```python
from build123d import *

# Parameters (mm, degrees)
SZKIC1_R                    = 6
SZKIC1_R_2                  = 3.5
DODANIE_WYCI_GNI_CIE1_DEPTH = 40
ZAOKR_GLENIE1_R             = 0.5
ZAOKR_GLENIE2_R             = 0.5


with BuildPart() as part:
    # Szkic1 → Dodanie-wyciągnięcie1 (new body)
    with BuildSketch(Plane.XY):
        Circle(SZKIC1_R)
        Circle(SZKIC1_R_2, mode=Mode.SUBTRACT)
    extrude(amount=-DODANIE_WYCI_GNI_CIE1_DEPTH)

    # Zaokrąglenie1
    zaokr_glenie1_edges = [part.edges().sort_by_distance(p)[0] for p in [
        (-6, 0, 0),
        (-6, 0, -40),
    ]]
    fillet(zaokr_glenie1_edges, radius=ZAOKR_GLENIE1_R)

    # Zaokrąglenie2
    zaokr_glenie2_edges = [part.edges().sort_by_distance(p)[0] for p in [
        (-3.5, 0, -40),
        (-3.5, 0, 0),
    ]]
    fillet(zaokr_glenie2_edges, radius=ZAOKR_GLENIE2_R)


solid = part.part
```
CAD build for the part. Positions are in the model's coordinates, mm. Give positions to 0.01 mm unless a question says otherwise; leave off trailing zeros. Loops run counter-clockwise (first coordinate to the right, second up) from the corner with the lowest first, then second, coordinate; pieces in that order, holes last. Notation, with made-up numbers: (13, 36.5) - (29, 36.5) arc R21 ccw to (29, 41.5) - close; hole circle Ø1 at (68.25, 73). An arc over 180 degrees is marked (long way). Put each result on its own line as item: value.
Q1. Mould opens along Y. For faces 1 (the face through (3.233, -1.341, -19.727)), 2 (the face through (-4, -2, -40)), 3 (the face through (-6, 0, -20)) say: pulls with the +Y half, pulls with the -Y half, needs draft (parallel to the pull), parting line crosses it, or undercut.
Filled in:
face 1: undercut
face 2: needs draft
face 3: parting line crosses it
Q2. Slice it at A-A (x = 0). Give the cut face in (y, z).
Filled in:
outline: (-6, -39.5) arc R0.5 ccw to (-5.5, -40) - (-4, -40) arc R0.5 ccw to (-3.5, -39.5) - (-3.5, -0.5) arc R0.5 ccw to (-4, 0) - (-5.5, 0) arc R0.5 ccw to (-6, -0.5) - close; (3.5, -39.5) arc R0.5 ccw to (4, -40) - (5.5, -40) arc R0.5 ccw to (6, -39.5) - (6, -0.5) arc R0.5 ccw to (5.5, 0) - (4, 0) arc R0.5 ccw to (3.5, -0.5) - close
Q3. Flat gauge pins, fed straight in: pin 1 (1 mm diameter, centred on y = -4, z = -15.5, fed in from +X); pin 2 (1.5 mm diameter, centred on x = 1, y = 2.5, fed in from +Z); pin 3 (2 mm diameter, centred on y = -1.5, z = -19, fed in from +X); pin 4 (4 mm diameter, centred on x = -3.5, z = -25, fed in from -Y). Where does each tip first touch, or does it go through?
Filled in:
pin 1: stops at x = 4.87
pin 2: passes through
pin 3: stops at x = 5.98
pin 4: stops at y = -5.81
Q4. Slice it at C-C (z = -10.5). Give the cut face in (x, y).
Filled in:
outline: circle Ø12 at (0, 0); hole circle Ø7 at (0, 0)
Q5. Probe line 1 along Y through (x, z) = (0, -27); line 2 along X through (y, z) = (0.25, -12.5); line 3 along Y through (x, z) = (-1.5, -11). List the from-to ranges inside material, lowest first.
Filled in:
line 1: y = -6 to -3.5, 3.5 to 6
line 2: x = -5.99 to -3.49, 3.49 to 5.99
line 3: y = -5.81 to -3.16, 3.16 to 5.81
